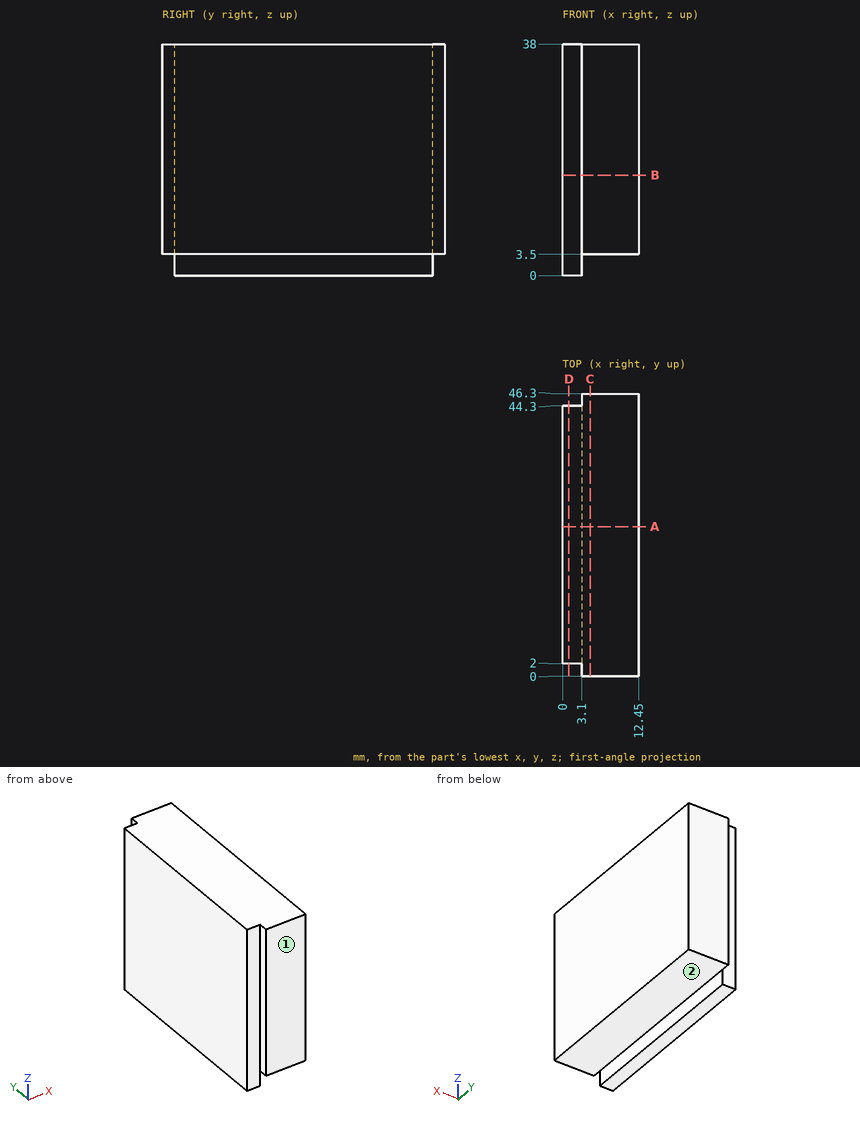
The drawing under review shows one solid part. Ordinate dimensions are in mm from its lowest x, y, z. A direction names the side the tool comes from. Coordinates: 2 decimals unless noted, no trailing zeros. Write each loop counter-clockwise with the first axis right and the second up, starting at its lowest first coordinate (ties: lowest second). Pieces come first, ordered by that corner, then holes. Notation, with made-up numbers: (24.5, 49.25) - (36.5, 49.25) arc R21 cw to (36.5, 67.25) - close; hole circle Ø8 at (26.5, 55.5). An arc over 180 degrees is marked (long way). Use one line per item in the form item = value.
Q1. Consider section C-C (x = 4.5). Write out the cut boundary in (y, z).
Taken from the geometry:
outline = (0, 3.5) - (46.3, 3.5) - (46.3, 38) - (0, 38) - close
Q2. Insertion check: pin 1 Ø1.8 at (y, z) = (22.5, 1) entering from +X; pin 2 Ø0.6 at (y, z) = (45.5, 16.5) entering from -X; pin 3 Ø4 at (x, y) = (6, 29.5) entering from -Z. Each pin has a flat end and moves straight along its axis. Give the tip position at first contact, or say it passes through.
Taken from the geometry:
pin_1 = 3.1
pin_2 = 3.1
pin_3 = 3.5
Q3. Consider section B-B (z = 16.5). Write out the cut boundary in (x, y), plus the area to 3 significant figures.
Taken from the geometry:
outline = (0, 2) - (3.1, 2) - (3.1, 0) - (12.45, 0) - (12.45, 46.3) - (3.1, 46.3) - (3.1, 44.3) - (0, 44.3) - close
area = 564 mm^2
Q4. For probe 1 along Z at (x, y) = (4.5, 13); probe 2 along Y at (x, z) = (3, 7), list the stretches that pass through material, from the lowest coordinate up.
Taken from the geometry:
probe_1 = 3.5 to 38
probe_2 = 2 to 44.3
Q5. Consider section A-A (y = 24.5). Write out the cut boundary in (x, z).
Taken from the geometry:
outline = (0, 0) - (3.1, 0) - (3.1, 3.5) - (12.45, 3.5) - (12.45, 38) - (0, 38) - close
Q6. Consider section D-D (x = 1). Write out the cut boundary in (y, z).
Taken from the geometry:
outline = (2, 0) - (44.3, 0) - (44.3, 38) - (2, 38) - close
Q7. Machinability: for the marked faces 1 and 2, which of the approach directions +Z, -Z, +X, -X, +Y, -Y give a long, thin tool a straight path to every point of the face, cutting with its end or side? Answer none if there is none.
Taken from the geometry:
face_1 = +Z, -Z, +X, -X, -Y
face_2 = -Z, +X, +Y, -Y
